CAD build for the part. Positions are in the model's coordinates, mm. Round coordinates to 2 decimals unless told otherwise and drop trailing zeros. Write each question's results on one line, items separated by ' | '. Start each with the question number.
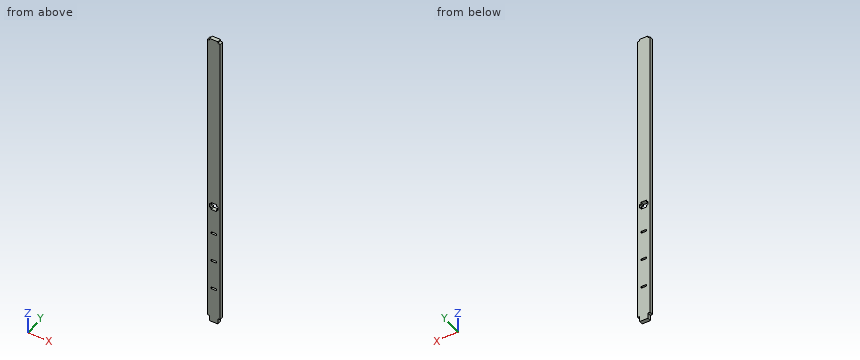
```python
from build123d import *

# Parameters (mm, degrees)
F1_DEPTH      = 3.175
F2_W          = 13.97
F2_H          = 3.175
F3_DEPTH      = 3.175
F3_DEPTH_BACK = 3.175
F4_W          = 13.97
F4_H          = 6.35
F5_DEPTH      = 6.35
F6_W          = 8.89
F6_H          = 3.175
F7_DEPTH      = 6.35
F8_W          = 8.89
F8_H          = 3.175
F9_DEPTH      = 6.35


with BuildPart() as f1:
    # F0 (on Front) → F1 (new body, symmetric)
    with BuildSketch(Plane.XZ):
        Polygon((-10.668, 508), (-10.668, 0), (-6.985, 0), (-6.985, -9.525), (6.985, -9.525), (6.985, 0), (10.668, 0), (10.668, 508), align=None)
    extrude(amount=F1_DEPTH, both=True)

    # F2 (on Front) → F3 (join, two sides)
    with BuildSketch(Plane.XZ) as f3_sk:
        with Locations((0, 509.5875)):
            Rectangle(F2_W, F2_H)
    extrude(amount=F3_DEPTH)
    extrude(f3_sk.sketch, amount=-F3_DEPTH_BACK)

    # F4 (on face) → F5 (cut, through all)
    with BuildSketch(Plane.XZ.offset(3.175)):
        with Locations((0, 203.2)):
            Rectangle(F4_W, F4_H)
    extrude(amount=-F5_DEPTH, mode=Mode.SUBTRACT)

    # F6 (on face) → F7 (cut, through all)
    with BuildSketch(Plane.XZ.offset(3.175)):
        with Locations((0, 207.9625)):
            Rectangle(F6_W, F6_H)
        with Locations((0, 198.4375)):
            Rectangle(F6_W, F6_H)
    extrude(amount=-F7_DEPTH, mode=Mode.SUBTRACT)

    # F8 (on face) → F9 (cut, through all)
    with BuildSketch(Plane.XZ.offset(3.175)):
        with Locations((0, 52.3875)):
            Rectangle(F8_W, F8_H)
        with Locations((0, 103.1875)):
            Rectangle(F8_W, F8_H)
        with Locations((0, 153.9875)):
            Rectangle(F8_W, F8_H)
    extrude(amount=-F9_DEPTH, mode=Mode.SUBTRACT)


solid = f1.part
```
1) Drop flat-ended pins along their axis: pin 1 Ø1.8 at (x, y) = (-8, 1.5) entering from +Z; pin 2 Ø3 at (y, z) = (-1, -5) entering from -X (3 decimals). Give the stop position or say it passes through.
2) Wall check: line 1 along Z through (x, y) = (1.75, 2.75) (3 decimals); line 2 along Z through (x, y) = (-4.5, 2.75) (3 decimals); line 3 along Z through (x, y) = (-9, -2). Give the ranges that are in metal, low to high. Write a range as from..to.
3) Saw through at A-A, the plane y = -1.25. State how many separate pieces and enclosed holes the cut face has, plus the area to 3 significant figures.
Filled sheet:
1) pin 1: stops at z = 508 | pin 2: stops at x = -6.985
2) line 1: z = -9.525..50.8, 53.975..101.6, 104.775..152.4, 155.575..196.85, 209.55..511.175 | line 2: z = -9.525..200.025, 206.375..511.175 | line 3: z = 0..508
3) separate pieces: 1 | enclosed holes: 4 | area: 10,800 mm^2
